from build123d import *

# Parameters (mm, degrees)
BOSS_EXTRUDE2_DEPTH = 25
SKETCH1_4_W         = 25
SKETCH1_4_H         = 400
BOSS_EXTRUDE3_DEPTH = 125
FILLET1_R           = 40
SKETCH2_R           = 20
CUT_EXTRUDE1_DEPTH  = 729.010988928
FILLET2_R           = 40
SKETCH3_R           = 7.94
CUT_EXTRUDE2_DEPTH  = 712.512473538


with BuildPart() as part:
    # Sketch1 → Boss-Extrude2 (new body)
    with BuildSketch(Plane(origin=(0, 0, 0), x_dir=(1, 0, 0), z_dir=(0, 1, 0))):
        Polygon((25, 400), (25, 0), (150, 0), (150, 200), (250, 300), (550, 300), (550, 400), align=None)
        with BuildLine():
            Line((550, 300), (550, 400))
            ThreePointArc((550, 400), (600, 350), (550, 300))
        make_face()
    extrude(amount=BOSS_EXTRUDE2_DEPTH)

    # Sketch1_4 → Boss-Extrude3 (add)
    with BuildSketch(Plane(origin=(0, 0, 0), x_dir=(1, 0, 0), z_dir=(0, 1, 0))):
        with Locations((12.5, 200)):
            Rectangle(SKETCH1_4_W, SKETCH1_4_H)
    extrude(amount=BOSS_EXTRUDE3_DEPTH)

    # Fillet1
    fillet1_edges = [part.edges().sort_by_distance(p)[0] for p in [
        (150, 12.5, 0),
    ]]
    fillet(fillet1_edges, radius=FILLET1_R)

    # Sketch2 → Cut-Extrude1 (cut, through all)
    with BuildSketch(Plane(origin=(0, 25, 0), x_dir=(1, 0, 0), z_dir=(0, 1, 0))):
        with Locations(Location((550, 350, 0), (0, 0, 270))):
            Circle(SKETCH2_R)
        with Locations(Location((125, 300, 0), (0, 0, 270))):
            Circle(SKETCH2_R)
    extrude(amount=-CUT_EXTRUDE1_DEPTH, mode=Mode.SUBTRACT)

    # Fillet2
    fillet2_edges = [part.edges().sort_by_distance(p)[0] for p in [
        (12.5, 125, -400),
        (12.5, 125, 0),
    ]]
    fillet(fillet2_edges, radius=FILLET2_R)

    # Sketch3 → Cut-Extrude2 (cut, through all)
    with BuildSketch(Plane(origin=(25, 0, 0), x_dir=(0, 0, -1), z_dir=(1, 0, 0))):
        with Locations((40, 85)):
            Circle(SKETCH3_R)
        with Locations(Location((360, 85, 0), (0, 0, 180))):
            Circle(SKETCH3_R)
    extrude(amount=-CUT_EXTRUDE2_DEPTH, mode=Mode.SUBTRACT)


solid = part.part
The model under review builds one solid part; all positions refer to its coordinate system, in mm. A direction names the side the tool comes from. Round coordinates to 2 decimals unless told otherwise and drop trailing zeros. Write each loop counter-clockwise with the first axis right and the second up, starting at its lowest first coordinate (ties: lowest second). Pieces come first, ordered by that corner, then holes. Notation, with made-up numbers: (50, 24.5) -> (66, 24.5) arc R29 cw to (66, 50.5) -> close; hole circle Ø3 at (-39.5, 53). An arc over 180 degrees is marked (long way). Answer as a JSON object with one key per item and string values.
1. We need section D-D on y = 59. State the section outline as (x, z) points.
Results found:
{"outline": "(0, -400) -> (25, -400) -> (25, 0) -> (0, 0) -> close"}
2. We need section C-C on x = 380. State the section outline as (y, z) points.
Results found:
{"outline": "(0, -400) -> (25, -400) -> (25, -300) -> (0, -300) -> close"}
3. Clearance check with flat-ended pins moving along their axes: pin 1 (3 mm diameter, centred on y = 27, z = -274.5, fed in from +X); pin 2 (20 mm diameter, centred on y = 7, z = -109, fed in from +X); pin 3 (2 mm diameter, centred on x = 161.5, z = -294.5, fed in from +Y); pin 4 (1.5 mm diameter, centred on x = 417.5, z = -315.5, fed in from -Y). State where each tip first meets the part, or that it passes through.
Results found:
{"pin 1": "stops at x = 25", "pin 2": "stops at x = 150", "pin 3": "stops at y = 25", "pin 4": "stops at y = 0"}
4. We need section A-A on x = 125. State the section outline as (y, z) points.
Results found:
{"outline": "(0, -400) -> (25, -400) -> (25, -320) -> (0, -320) -> close; (0, -280) -> (25, -280) -> (25, -2.92) -> (0, -2.92) -> close"}
5. We need section B-B on z = -186.5. State the section outline as (x, y) points, and give its area (3 significant figures).
Results found:
{"outline": "(0, 0) -> (150, 0) -> (150, 25) -> (25, 25) -> (25, 125) -> (0, 125) -> close", "area": "6,250 mm^2"}
6. To check wall thickness, follow line 1 along X through (y, z) = (16.5, -350); line 2 along Y through (x, z) = (17, -360); line 3 along X through (y, z) = (102, -219). State the ranges of each line that lie inside material, in increasing order.
Results found:
{"line 1": "x = 0 to 530, 570 to 600", "line 2": "y = 0 to 77.06, 92.94 to 125", "line 3": "x = 0 to 25"}
7. Machinability: for faces 1 (the face through (25, 74, -197)), 2 (the face through (117.34, 12.675, -281.525)), 3 (the face through (398, 12, -300)), which of the approach directions +Z, -Z, +X, -X, +Y, -Y give a long, thin tool a straight path to every point of the face, cutting with its end or side? Answer none if there is none.
Results found:
{"face 1": "+Z, -Z, +X, +Y", "face 2": "+Y, -Y", "face 3": "+Z, +X, +Y, -Y"}
8. The part is to be moulded in two halves that separate along Z. For faces 4 (the face through (42, 23, 0)), 5 (the face through (150, 12, -119)), 6 (the face through (12.675, 84.651, -367.932)), say which applies: pulls with the +Z half, pulls with the -Z half, needs draft (parallel to the pull), parting line crosses it, or undercut.
Results found:
{"face 4": "pulls with the +Z half", "face 5": "needs draft", "face 6": "undercut"}
